Check sheet for the modelled part. Datum: model origin and axes. Units: mm. A direction names the side the tool comes from. Round coordinates to 2 decimals unless told otherwise and drop trailing zeros. Order: outer loops, then holes, each group sorted by start corner. A loop starts at its lowest first (then second) coordinate and runs counter-clockwise, first axis right, second up.
Q1. Cross-section at B-B on y = 264.5. Record the cut outline in (x, z) (3 decimals), then the cut area to 3 significant figures.
Q2. Scan lines: probe 1 along Z at (x, y) = (136, 493); probe 2 along X at (y, z) = (507, 121.5) (3 decimals); probe 3 along Z at (x, y) = (20, 351.5). Record each from-to range of solid material in increasing order.
Q3. Cross-section at C-C on z = 217.5. Record the cut outline in (x, y) (3 decimals).
Q4. Set-up check for faces 1 (the flat face through (178, 0, 268)), 2 (the flat face through (19.16, 263.59, 253.37)): record each of +Z, -Z, +X, -X, +Y, -Y from which the full face is reachable in a straight line by a thin tool's end or side.
Q5. Mould release check, pull along Z, two halves, no side actions. Record for faces 3 (the flat face through (0, 264, 135)), 4 (the flat face through (227, 271, 0)), 5 (the flat face through (18.845, 263.592, 20.175)): +Z half, -Z half, draft (parallel to the pull), parting line (faces both ways), or undercut.
Q6. Cross-section at A-A on x = 158.5. Record the cut outline in (y, z), then the cut area to 3 significant figures.
from build123d import *

# Parameters (mm, degrees)
F0_W     = 460.375
F0_H     = 534.67
F1_DEPTH = 273.2278
F3_DEPTH = 536.956


# Not quite as in the source:
# - a feature names something its author has since deleted; it is built from what else it names


with BuildPart() as f1:
    # F0 (on Top) → F1 (new body)
    with BuildSketch(Plane.XY):
        with Locations((230.1875, 267.335)):
            Rectangle(F0_W, F0_H)
    extrude(amount=F1_DEPTH)

    # F2 (on face) → F3 (cut)
    with BuildSketch(Plane.XZ):
        Polygon((452.7307115978, 241.8399496412), (430.0117425975, 264.584589793), (30.3632574025, 264.584589793), (7.6442884022, 241.8399496412), (7.6442884022, 31.3878503588), (30.3632574025, 8.643210207), (427.9011, 8.643210207), (452.7307115978, 32.4993), align=None)
    extrude(amount=-F3_DEPTH, mode=Mode.SUBTRACT)


solid = f1.part
Results found:
1. outline: (0, 0) - (460.375, 0) - (460.375, 273.228) - (0, 273.228) - close; hole (7.644, 31.388) - (30.363, 8.643) - (427.901, 8.643) - (452.731, 32.499) - (452.731, 241.84) - (430.012, 264.585) - (30.363, 264.585) - (7.644, 241.84) - close
1. area: 12,900 mm2
2. probe 1: z = 0 to 8.64, 264.58 to 273.23
2. probe 2: x = 0 to 7.644, 452.731 to 460.375
2. probe 3: z = 0 to 19.02, 254.21 to 273.23
3. outline: (0, 0) - (7.644, 0) - (7.644, 534.67) - (0, 534.67) - close; (452.731, 0) - (460.375, 0) - (460.375, 534.67) - (452.731, 534.67) - close
4. face 1: +Z, -Z, +X, -X, -Y
4. face 2: +Y, -Y
5. face 3: draft
5. face 4: -Z half
5. face 5: undercut
6. outline: (0, 0) - (534.67, 0) - (534.67, 8.64) - (0, 8.64) - close; (0, 264.58) - (534.67, 264.58) - (534.67, 273.23) - (0, 273.23) - close
6. area: 9,240 mm2
